from build123d import *

# Parameters (mm, degrees)
SKETCH1_W           = 80
SKETCH1_H           = 64
BOSS_EXTRUDE1_DEPTH = 20
SHELL1_T            = 4
SKETCH2_W           = 4
SKETCH2_H           = 4
SKETCH2_W_2         = 11
CUT_EXTRUDE1_DEPTH  = 20
SKETCH4_W           = 72
SKETCH4_H           = 3
BOSS_EXTRUDE3_DEPTH = 10
SKETCH3_W           = 72
SKETCH3_H           = 3
BOSS_EXTRUDE2_DEPTH = 10
SKETCH6_W           = 7
SKETCH6_H           = 66
CUT_EXTRUDE2_DEPTH  = 3


with BuildPart() as part:
    # Sketch1 → Boss-Extrude1 (new body)
    with BuildSketch(Plane(origin=(0, 0, 0), x_dir=(1, 0, 0), z_dir=(0, 1, 0))):
        Rectangle(SKETCH1_W, SKETCH1_H)
    extrude(amount=BOSS_EXTRUDE1_DEPTH)

    # Shell1
    shell1_openings = [part.faces().sort_by_distance(p)[0] for p in [
        (0, 20, 0),
    ]]
    offset(amount=SHELL1_T, openings=shell1_openings, kind=Kind.INTERSECTION)

    # Sketch2 → Cut-Extrude1 (cut)
    with BuildSketch(Plane(origin=(0, 20, 0), x_dir=(1, 0, 0), z_dir=(0, 1, 0))):
        with Locations((-42, -23)):
            Rectangle(SKETCH2_W, SKETCH2_H)
        with Locations((34.5, -34)):
            Rectangle(SKETCH2_W_2, SKETCH2_H)
        with Locations((42, -21.5)):
            Rectangle(SKETCH2_W, SKETCH2_H)
        with Locations((30, 34)):
            Rectangle(SKETCH2_W, SKETCH2_H)
        with Locations((-33, 34)):
            Rectangle(SKETCH2_W, SKETCH2_H)
    extrude(amount=-CUT_EXTRUDE1_DEPTH, mode=Mode.SUBTRACT)

    # Sketch4 → Boss-Extrude3 (add)
    with BuildSketch(Plane.ZY.offset(44)):
        with Locations((0, -2.5)):
            Rectangle(SKETCH4_W, SKETCH4_H)
    extrude(amount=BOSS_EXTRUDE3_DEPTH)

    # Sketch3 → Boss-Extrude2 (add)
    with BuildSketch(Plane(origin=(44, 0, 0), x_dir=(0, 0, -1), z_dir=(1, 0, 0))):
        with Locations((0, -2.5)):
            Rectangle(SKETCH3_W, SKETCH3_H)
    extrude(amount=BOSS_EXTRUDE2_DEPTH)

    # Sketch6 → Cut-Extrude2 (cut)
    with BuildSketch(Plane(origin=(0, -1, 0), x_dir=(1, 0, 0), z_dir=(0, 1, 0))):
        with Locations((-47.5, 0)):
            Rectangle(SKETCH6_W, SKETCH6_H)
        with Locations((47.5, 0)):
            Rectangle(SKETCH6_W, SKETCH6_H)
    extrude(amount=-CUT_EXTRUDE2_DEPTH, mode=Mode.SUBTRACT)


solid = part.part
The model under review builds one solid part; all positions refer to its coordinate system, in mm. A direction names the side the tool comes from. Round coordinates to 2 decimals unless told otherwise and drop trailing zeros. Write each loop counter-clockwise with the first axis right and the second up, starting at its lowest first coordinate (ties: lowest second). Pieces come first, ordered by that corner, then holes. Notation, with made-up numbers: (-29.75, 16.5) -> (-7.75, 16.5) arc R10 ccw to (-7.75, 27.5) -> close; hole circle Ø4 at (6.5, -34). An arc over 180 degrees is marked (long way). Answer as a JSON object with one key per item and string values.
1. Clearance check with flat-ended pins moving along their axes: pin 1 (1.2 mm diameter, centred on y = 6.5, z = -34.5, fed in from -X); pin 2 (1.2 mm diameter, centred on y = 6.5, z = -34, fed in from +X); pin 3 (6.5 mm diameter, centred on x = 36.5, y = 10, fed in from +Z). State where each tip first meets the part, or that it passes through.
Results found:
{"pin 1": "stops at x = -44", "pin 2": "stops at x = 44", "pin 3": "stops at z = -32"}
2. We need section B-B on z = -7. State the section outline as (x, y) points.
Results found:
{"outline": "(-54, -4) -> (-51, -4) -> (-51, -1) -> (-54, -1) -> close; (-44, -4) -> (44, -4) -> (44, 20) -> (40, 20) -> (40, 0) -> (-40, 0) -> (-40, 20) -> (-44, 20) -> close; (51, -4) -> (54, -4) -> (54, -1) -> (51, -1) -> close"}
3. The part is to be moulded in two halves that separate along X. For faces 4 (the face through (-54, -2, -1)), 5 (the face through (-16, 20, 33)), 6 (the face through (-51, -2, 0)), say which applies: pulls with the +X half, pulls with the -X half, needs draft (parallel to the pull), parting line crosses it, or undercut.
Results found:
{"face 4": "pulls with the -X half", "face 5": "needs draft", "face 6": "undercut"}
4. To check wall thickness, follow line 1 along Z through (x, y) = (-40.5, 5.5); line 2 along X through (y, z) = (16, -10); line 3 along X through (y, z) = (6.25, -33). State the ranges of each line that lie inside material, in increasing order.
Results found:
{"line 1": "z = -36 to 21, 25 to 36", "line 2": "x = -44 to -40, 40 to 44", "line 3": "x = -44 to -35, -31 to 28, 32 to 44"}
5. We need section C-C on x = 25. State the section outline as (y, z) points, and give its area (3 significant figures).
Results found:
{"outline": "(-4, -36) -> (20, -36) -> (20, -32) -> (0, -32) -> (0, 32) -> (20, 32) -> (20, 36) -> (-4, 36) -> close", "area": "448 mm^2"}
6. We need section A-A on y = 17.75. State the section outline as (x, z) points, and give its area (3 significant figures).
Results found:
{"outline": "(-44, -36) -> (-35, -36) -> (-35, -32) -> (-40, -32) -> (-40, 21) -> (-44, 21) -> close; (-44, 25) -> (-40, 25) -> (-40, 32) -> (29, 32) -> (29, 36) -> (-44, 36) -> close; (-31, -36) -> (28, -36) -> (28, -32) -> (-31, -32) -> close; (32, -36) -> (44, -36) -> (44, 19.5) -> (40, 19.5) -> (40, -32) -> (32, -32) -> close; (40, 23.5) -> (44, 23.5) -> (44, 36) -> (40, 36) -> close", "area": "1,110 mm^2"}
7. Machinability: for faces 1 (the face through (32, 10, -34)), 2 (the face through (42, 10, 23.5)), 3 (the face through (47, -2, -33)), which of the approach directions +Z, -Z, +X, -X, +Y, -Y give a long, thin tool a straight path to every point of the face, cutting with its end or side? Answer none if there is none.
Results found:
{"face 1": "+Z, -Z, +Y", "face 2": "+X, -X, +Y", "face 3": "+Y, -Y"}
